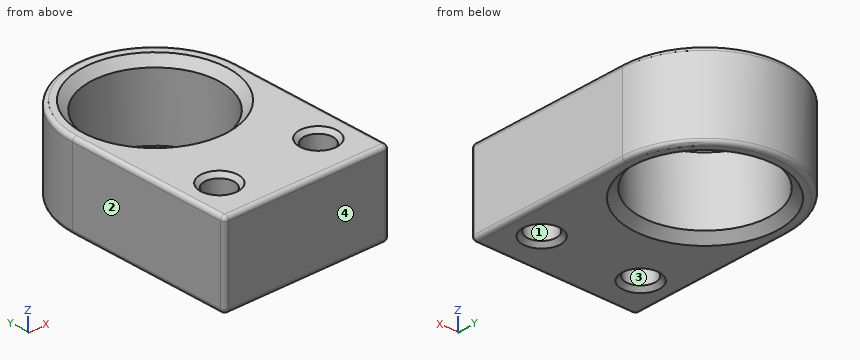
```python
from build123d import *

# Parameters (mm, degrees)
SKETCH_1_W      = 20
SKETCH_1_H      = 10
SKETCH_1_R      = 1.75
EXTRUDE_1_DEPTH = 10
SKETCH_2_R      = 7.75
EXTRUDE_2_DEPTH = 10
CHAMFER_1_SIZE  = 1
CHAMFER_2_SIZE  = 0.5
FILLET_1_R      = 0.5


with BuildPart() as part:
    # 草图1 → 凸台-拉伸1 (new body)
    with BuildSketch(Plane.XY):
        Rectangle(SKETCH_1_W, SKETCH_1_H)
        with Locations((-6, 0)):
            Circle(SKETCH_1_R, mode=Mode.SUBTRACT)
        with Locations((6, 0)):
            Circle(SKETCH_1_R, mode=Mode.SUBTRACT)
    extrude(amount=EXTRUDE_1_DEPTH)

    # 草图2 → 凸台-拉伸2 (add)
    with BuildSketch(Plane.XY.offset(10)):
        with BuildLine():
            Line((-10, 15), (-10, 5))
            Line((-10, 5), (10, 5))
            Line((10, 5), (10, 15))
            ThreePointArc((10, 15), (0, 25), (-10, 15))
        make_face()
        with Locations((0, 15)):
            Circle(SKETCH_2_R, mode=Mode.SUBTRACT)
    extrude(amount=-EXTRUDE_2_DEPTH)

    # 倒角1
    chamfer_1_edges = [part.edges().sort_by_distance(p)[0] for p in [
        (-7.75, 15, 10),
        (-7.75, 15, 0),
    ]]
    chamfer(chamfer_1_edges, length=CHAMFER_1_SIZE)

    # 倒角2
    chamfer_2_edges = [part.edges().sort_by_distance(p)[0] for p in [
        (-7.75, 0, 0),
        (-7.75, 0, 10),
        (4.25, 0, 0),
        (4.25, 0, 10),
    ]]
    chamfer(chamfer_2_edges, length=CHAMFER_2_SIZE)

    # 圆角1
    fillet_1_edges = [part.edges().sort_by_distance(p)[0] for p in [
        (-10, 5, 10),
        (0, -5, 10),
        (0, 25, 0),
        (0, 25, 10),
        (10, 5, 10),
        (0, -5, 0),
        (-10, 5, 0),
        (10, 5, 0),
        (10, -5, 5),
        (-10, -5, 5),
    ]]
    fillet(fillet_1_edges, radius=FILLET_1_R)


solid = part.part
```
Design review of the part built by this model. Coordinates are the model's own, in mm. Face numbers are marked on the shaded views. Round coordinates to 2 decimals unless told otherwise and drop trailing zeros. Order: outer loops, then holes, each group sorted by start corner. A loop starts at its lowest first (then second) coordinate and runs counter-clockwise, first axis right, second up. Notation, with made-up numbers: (59.5, 53) - (70.5, 53) arc R14 ccw to (70.5, 65) - close; hole circle Ø10 at (15.5, -19.75). An arc over 180 degrees is marked (long way). Return JSON: item names as keys, results as strings.
Q1. Consider section C-C on x = 0. Write out the cut boundary in (y, z).
Computed values:
{"outline": "(-5, 0.5) arc R0.5 ccw to (-4.5, 0) - (6.25, 0) - (7.25, 1) - (7.25, 9) - (6.25, 10) - (-4.5, 10) arc R0.5 ccw to (-5, 9.5) - close; (22.75, 1) - (23.75, 0) - (24.5, 0) arc R0.5 ccw to (25, 0.5) - (25, 9.5) arc R0.5 ccw to (24.5, 10) - (23.75, 10) - (22.75, 9) - close"}
Q2. The part is to be moulded in two halves that separate along X. For the marked faces 1, 2, 3 and 4, say which applies: pulls with the +X half, pulls with the -X half, needs draft (parallel to the pull), parting line crosses it, or undercut.
Computed values:
{"face 1": "undercut", "face 2": "pulls with the -X half", "face 3": "undercut", "face 4": "needs draft"}
Q3. Consider section B-B on y = 0. Write out the cut boundary in (x, z).
Computed values:
{"outline": "(-10, 0.5) arc R0.5 ccw to (-9.5, 0) - (-8.25, 0) - (-7.75, 0.5) - (-7.75, 9.5) - (-8.25, 10) - (-9.5, 10) arc R0.5 ccw to (-10, 9.5) - close; (-4.25, 0.5) - (-3.75, 0) - (3.75, 0) - (4.25, 0.5) - (4.25, 9.5) - (3.75, 10) - (-3.75, 10) - (-4.25, 9.5) - close; (7.75, 0.5) - (8.25, 0) - (9.5, 0) arc R0.5 ccw to (10, 0.5) - (10, 9.5) arc R0.5 ccw to (9.5, 10) - (8.25, 10) - (7.75, 9.5) - close"}
Q4. Wall thickness on L1, parallel to X at y = 1.25, z = 8; L2, parallel to Y at x = 6, z = 6.5; L3, parallel to Y at x = -6.5, z = 6.75: over which ranges is each line inside the solid? List them lowest first. Write a range as [from, to].
Computed values:
{"L1": "x = [-10, -7.22], [-4.78, 4.78], [7.22, 10]", "L2": "y = [-5, -1.75], [1.75, 10.09], [19.91, 23]", "L3": "y = [-5, -1.68], [1.68, 10.78], [19.22, 22.6]"}
Q5. For pin 1 Ø3 at (x, y) = (6.5, 0.5) entering from +Z; pin 2 Ø3 at (x, y) = (-6, 0) entering from -Z; pin 3 Ø5 at (y, z) = (19.5, 9) entering from -X, all flat-tipped, find the tip position at first contact; note any pin that passes through.
Computed values:
{"pin 1": "stops at z = 9.96", "pin 2": "passes through", "pin 3": "stops at x = -9.8"}
Q6. Consider section A-A on z = 3.5. Write out the cut boundary in (x, y).
Computed values:
{"outline": "(-10, -4.5) arc R0.5 ccw to (-9.5, -5) - (9.5, -5) arc R0.5 ccw to (10, -4.5) - (10, 15) arc R10 ccw to (-10, 15) - close; hole circle Ø3.5 at (-6, 0); hole circle Ø15.5 at (0, 15); hole circle Ø3.5 at (6, 0)"}
Q7. Consider section D-D on x = 6. Give the number of separate pieces and of enclosed holes in the cut face, plus the area to 3 significant figures.
Computed values:
{"separate pieces": "3", "enclosed holes": "0", "area": "143 mm2"}
